from build123d import *

# Parameters (mm, degrees)
SKETCH1_W           = 76.2
SKETCH1_H           = 25.4
BOSS_EXTRUDE1_DEPTH = 12.7
SKETCH2_W           = 19.05
SKETCH2_H           = 6.35
CUT_EXTRUDE1_DEPTH  = 82.319677815
CUT_EXTRUDE2_DEPTH  = 3.175
FILLET1_R           = 1.27
CHAMFER1_SIZE       = 0.635
CHAMFER1_SIZE2      = 0.231121099


with BuildPart() as part:
    # Sketch1 → Boss-Extrude1 (new body)
    with BuildSketch(Plane(origin=(0, 0, 0), x_dir=(1, 0, 0), z_dir=(0, 1, 0))):
        with Locations((38.1, 12.7)):
            Rectangle(SKETCH1_W, SKETCH1_H)
    extrude(amount=BOSS_EXTRUDE1_DEPTH)

    # Sketch2 → Cut-Extrude1 (cut, through all)
    with BuildSketch(Plane(origin=(76.2, 0, 0), x_dir=(0, 0, -1), z_dir=(1, 0, 0))):
        with Locations((12.7, 6.35)):
            Rectangle(SKETCH2_W, SKETCH2_H)
    extrude(amount=-CUT_EXTRUDE1_DEPTH, mode=Mode.SUBTRACT)

    # Sketch3 → Cut-Extrude2 (cut)
    with BuildSketch(Plane(origin=(0, 12.7, 0), x_dir=(1, 0, 0), z_dir=(0, 1, 0))):
        with BuildLine():
            Line((12.573, 6.35), (63.627, 6.35))
            ThreePointArc((63.627, 6.35), (68.027325499, 8.172674501), (69.85, 12.573))
            Line((69.85, 12.573), (69.85, 12.827))
            ThreePointArc((69.85, 12.827), (68.027325499, 17.227325499), (63.627, 19.05))
            Line((63.627, 19.05), (12.573, 19.05))
            ThreePointArc((12.573, 19.05), (8.172674501, 17.227325499), (6.35, 12.827))
            Line((6.35, 12.827), (6.35, 12.573))
            ThreePointArc((6.35, 12.573), (8.172674501, 8.172674501), (12.573, 6.35))
        make_face()
    extrude(amount=-CUT_EXTRUDE2_DEPTH, mode=Mode.SUBTRACT)

    # Fillet1
    fillet1_edges = [part.edges().sort_by_distance(p)[0] for p in [
        (76.2, 12.7, -12.7),
        (38.1, 12.7, -25.4),
        (0, 12.7, -12.7),
        (38.1, 0, -25.4),
        (76.2, 0, -12.7),
        (38.1, 0, 0),
        (0, 0, -12.7),
        (0, 6.35, -25.4),
        (76.2, 6.35, -25.4),
        (76.2, 6.35, 0),
        (0, 6.35, 0),
        (38.1, 12.7, 0),
    ]]
    fillet(fillet1_edges, radius=FILLET1_R)

    # Chamfer1
    chamfer1_edges = [part.edges().sort_by_distance(p)[0] for p in [
        (68.027325499, 12.7, -17.227325499),
        (38.1, 12.7, -19.05),
        (8.172674501, 12.7, -17.227325499),
        (6.35, 12.7, -12.7),
        (8.172674501, 12.7, -8.172674501),
        (38.1, 12.7, -6.35),
        (68.027325499, 12.7, -8.172674501),
        (69.85, 12.7, -12.7),
    ]]
    chamfer1_side = [part.faces().sort_by_distance(p)[0] for p in [
        (74.158742896, 12.7, -12.7),
    ]]
    chamfer(chamfer1_edges, length=CHAMFER1_SIZE, length2=CHAMFER1_SIZE2, reference=chamfer1_side[0])


solid = part.part
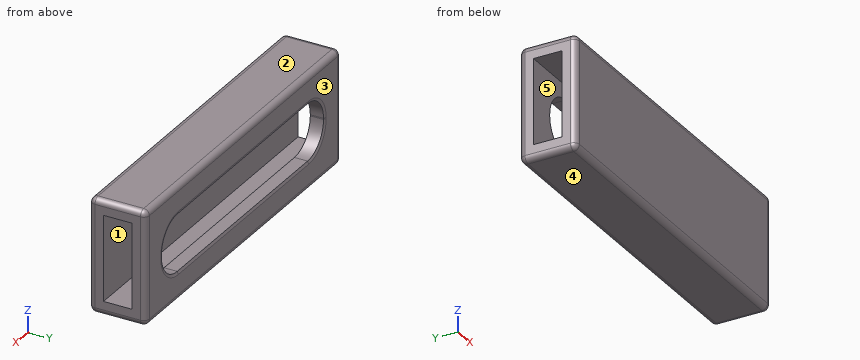
Input: part model. Units: mm. Frame: model coordinates. Face numbers are marked on the shaded views. A direction names the side the tool comes from. Coordinates: 2 decimals unless noted, no trailing zeros. Loops run counter-clockwise (first coordinate to the right, second up) from the corner with the lowest first, then second, coordinate; pieces in that order, holes last.
Q1. Material intervals for line 1 (Z direction, x = 53, y = 4.5) (3 decimals); line 2 (Y direction, x = 6, z = -15) (3 decimals); line 3 (Z direction, x = 17.5, y = 10), sorted ascending.
Q2. Set-up query: the marked faces 4 and 5. Return all of +Z, -Z, +X, -X, +Y, -Y with unobstructed straight access to the full face (end or side cutting, diameter ignored); none if empty.
Q3. Contact query for a flat-ended pin moving along its axis: pin 1 (10 mm diameter, centred on x = 14.5, z = -6.5, fed in from +Y). Output: stop coordinate, or through.
Q4. Cut plane D-D (z = -7.75). Give the number of separate pieces and of enclosed holes in the cut face, then the cut area to 3 significant figures.
Q5. Cut plane A-A (y = 8.5). Output: boundary loops of the cut face in (x, z) (3 decimals), then the cut area to 3 significant figures.
Q6. Draft query along Y for the marked faces 1, 2 and 3. Return one class per face: +Y half, -Y half, draft (parallel to the pull), parting line (faces both ways), or undercut.
Q7. Cut plane C-C (x = 20). Output: boundary loops of the cut face in (y, z) (3 decimals).
Q8. Cut plane B-B (z = -4.25). Output: boundary loops of the cut face in (x, y) (3 decimals).
Working result:
1. line 1: z = -25.4 to -22.225, -3.175 to 0
1. line 2: y = 0 to 3.175, 9.525 to 12.7
1. line 3: z = -25.4 to -19.05, -6.35 to 0
2. face 4: -Z, +X, -X, +Y, -Y
2. face 5: +X, -X
3. pin 1: stops at y = 12.7
4. separate pieces: 3
4. enclosed holes: 0
4. area: 295 mm2
5. outline: (0, -24.13) arc R1.27 ccw to (1.27, -25.4) - (74.93, -25.4) arc R1.27 ccw to (76.2, -24.13) - (76.2, -22.225) - (0, -22.225) - close; (0, -3.175) - (76.2, -3.175) - (76.2, -1.27) arc R1.27 ccw to (74.93, 0) - (1.27, 0) arc R1.27 ccw to (0, -1.27) - close
5. area: 482 mm2
6. face 1: undercut
6. face 2: draft
6. face 3: +Y half
7. outline: (0, -24.13) arc R1.27 ccw to (1.27, -25.4) - (11.43, -25.4) arc R1.27 ccw to (12.7, -24.13) - (12.7, -19.685) - (12.469, -19.05) - (9.525, -19.05) - (9.525, -22.225) - (3.175, -22.225) - (3.175, -3.175) - (9.525, -3.175) - (9.525, -6.35) - (12.469, -6.35) - (12.7, -5.715) - (12.7, -1.27) arc R1.27 ccw to (11.43, 0) - (1.27, 0) arc R1.27 ccw to (0, -1.27) - close
8. outline: (0, 1.27) arc R1.27 ccw to (1.27, 0) - (74.93, 0) arc R1.27 ccw to (76.2, 1.27) - (76.2, 3.175) - (0, 3.175) - close; (0, 9.525) - (76.2, 9.525) - (76.2, 11.43) arc R1.27 ccw to (74.93, 12.7) - (1.27, 12.7) arc R1.27 ccw to (0, 11.43) - close
